Study the drawing (mm; zero at the part's minimum x, y, z) and answer. Coordinates: 2 decimals unless noted, no trailing zeros. Order: outer loops, then holes, each group sorted by start corner. A loop starts at its lowest first (then second) coordinate and runs counter-clockwise, first axis right, second up. Notation, with made-up numbers: M 21,26 L 75,26 A31 cw 75,51 Z; hole C 20,64.25 d8. An arc over 180 degrees is marked long. Use a Markdown table: item, result. Add a question column.
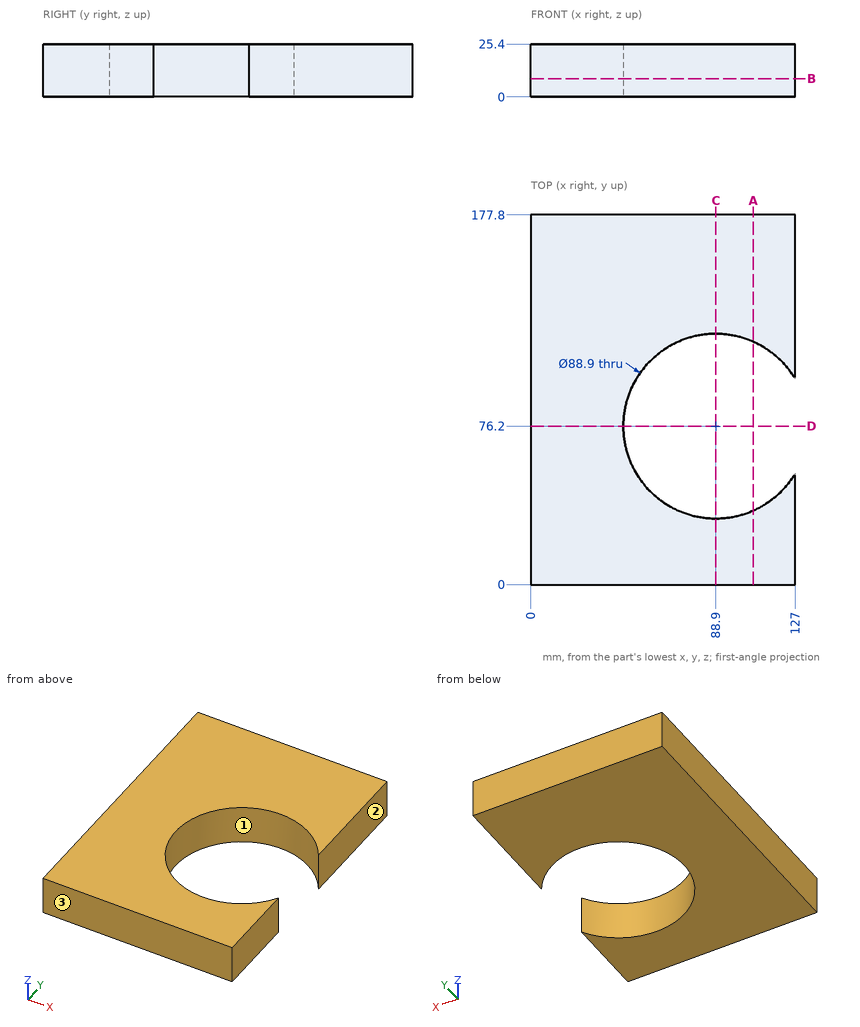
(1) A cutting plane is placed at B-B on z = 8.75. Write down the section's boundary in (x, y), plus the area to 3 significant figures.
(2) Straight lines are drawn through the part: line 1 (Y direction, x = 88.9, z = 18.25); line 2 (X direction, y = 76.2, z = 9); line 3 (Y direction, x = 68.5, z = 17.75). For each, find the intervals that lie inside material, in ascending order.
(3) A cutting plane is placed at C-C on x = 88.9. Write down the section's boundary in (y, z), plus the area to 3 significant figures.
(4) The mould has two halves that part along X. Classify the marked faces 1, 2 and 3: pulls with the +X half, pulls with the -X half, needs draft (parallel to the pull), parting line crosses it, or undercut.
(5) A cutting plane is placed at A-A on x = 107. Write down the section's boundary in (y, z).
(6) A cutting plane is placed at D-D on y = 76.2. Write down the section's boundary in (x, z), plus the area to 3 significant figures.
From the geometry:
| question | item | result |
|---|---|---|
| 1 | outline | M 0,0 L 127,0 L 127,53.3 A44.45 cw long 127,99.1 L 127,177.8 L 0,177.8 Z |
| 1 | area | 16,600 mm2 |
| 2 | line 1 | y = 0 to 31.75, 120.65 to 177.8 |
| 2 | line 2 | x = 0 to 44.45 |
| 2 | line 3 | y = 0 to 36.71, 115.69 to 177.8 |
| 3 | outline | M 0,0 L 31.75,0 L 31.75,25.4 L 0,25.4 Z; M 120.65,0 L 177.8,0 L 177.8,25.4 L 120.65,25.4 Z |
| 3 | area | 2,260 mm2 |
| 4 | face 1 | undercut |
| 4 | face 2 | pulls with the +X half |
| 4 | face 3 | needs draft |
| 5 | outline | M 0,0 L 35.6,0 L 35.6,25.4 L 0,25.4 Z; M 116.8,0 L 177.8,0 L 177.8,25.4 L 116.8,25.4 Z |
| 6 | outline | M 0,0 L 44.45,0 L 44.45,25.4 L 0,25.4 Z |
| 6 | area | 1,130 mm2 |
